```python
from build123d import *

# Parameters (mm, degrees)
SKETCH1_W           = 52
SKETCH1_H           = 53
BOSS_EXTRUDE1_DEPTH = 2
SKETCH2_W           = 48
SKETCH2_H           = 49
SKETCH2_W_2         = 44
SKETCH2_H_2         = 45
BOSS_EXTRUDE2_DEPTH = 5
CUT_EXTRUDE1_START  = -7
SKETCH3_W           = 4
SKETCH3_H           = 20
CUT_EXTRUDE1_DEPTH  = 7
FILLET1_R           = 2
SKETCH4_W           = 48
SKETCH4_H           = 2
CUT_EXTRUDE2_DEPTH  = 5


with BuildPart() as part:
    # Sketch1 → Boss-Extrude1 (new body)
    with BuildSketch(Plane.XY):
        with Locations((26, 26.5)):
            Rectangle(SKETCH1_W, SKETCH1_H)
    extrude(amount=BOSS_EXTRUDE1_DEPTH)

    # Sketch2 → Boss-Extrude2 (add)
    with BuildSketch(Plane.XY.offset(2)):
        with Locations((26, 26.5)):
            Rectangle(SKETCH2_W, SKETCH2_H)
        with Locations((26, 26.5)):
            Rectangle(SKETCH2_W_2, SKETCH2_H_2, mode=Mode.SUBTRACT)
    extrude(amount=BOSS_EXTRUDE2_DEPTH)

    # Sketch3 → Cut-Extrude1 (cut)
    with BuildSketch(Plane(origin=(0, 0, 0), x_dir=(-1, 0, 0), z_dir=(0, 0, -1)).offset(CUT_EXTRUDE1_START)):
        with Locations((-50, 25.5)):
            Rectangle(SKETCH3_W, SKETCH3_H)
    extrude(amount=CUT_EXTRUDE1_DEPTH, mode=Mode.SUBTRACT)

    # Fillet1
    fillet1_edges = [part.edges().sort_by_distance(p)[0] for p in [
        (48, 15.5, 1),
        (48, 35.5, 1),
    ]]
    fillet(fillet1_edges, radius=FILLET1_R)
    fillet1_2_edges = [part.edges().sort_by_distance(p)[0] for p in [
        (52, 15.5, 1),
        (52, 35.5, 1),
    ]]
    fillet(fillet1_2_edges, radius=FILLET1_R - 0.0001)  # a hair under: the kernel refuses the full size

    # Sketch4 → Cut-Extrude2 (cut)
    with BuildSketch(Plane.XY.offset(7)):
        with Locations((26, 3)):
            Rectangle(SKETCH4_W, SKETCH4_H)
    extrude(amount=-CUT_EXTRUDE2_DEPTH, mode=Mode.SUBTRACT)


solid = part.part
```
Verification items for the finished model (mm, model axes). A direction names the side the tool comes from. Round coordinates to 2 decimals unless told otherwise and drop trailing zeros. Order: outer loops, then holes, each group sorted by start corner. A loop starts at its lowest first (then second) coordinate and runs counter-clockwise, first axis right, second up. Notation, with made-up numbers: (25, -11) -> (57, -11) arc R6 cw to (57, -4) -> close; hole circle Ø2 at (-39.75, 26). An arc over 180 degrees is marked (long way). Put each result on its own line as item: value. Start each with the question number.
(1) Section check D-D (y = 29). Enter the section's corners in (x, z).
(2) Section check A-A (z = 5.25). Enter the section's corners in (x, y).
(3) Draft check along X on faces 5 (the face through (26, 49, 4)), 6 (the face through (26, 21, 2)), 7 (the face through (26, 51, 4)), 8 (the face through (0, 26, 1)). Enter one of: +X half, -X half, draft (parallel to the pull), parting line (faces both ways), or undercut.
(4) Section check B-B (y = 47). Enter the section's corners in (x, z).
(5) Material ranges on line 1 along X through (y, z) = (6.5, 4.5); line 2 along Z through (x, y) = (12.5, 3); line 3 along Y through (x, z) = (47, 5.5), recorded low to high.
(6) Section check C-C (x = 24). Enter the section's corners in (y, z).
(7) Tool access check on faces 1 (the face through (48, 42, 4)), 2 (the face through (2, 27, 4)), 3 (the face through (51.4, 36.07, 0.99)), 4 (the face through (49, 4, 5)). Record the directions out of +Z, -Z, +X, -X, +Y, -Y that give a thin tool (end or side, any length) a straight path to the whole face; none if there is none.
(8) Depth check by flat-ended pin: pin 1 Ø1 at (x, z) = (49, 3.5) entering from -Y; pin 2 Ø1.6 at (x, z) = (49, 4.5) entering from +Y; pin 3 Ø1.5 at (y, z) = (18.5, 4.5) entering from -X. Enter the tip coordinate at first touch or a pass-through.
Completed:
1. outline: (0, 0) -> (48, 0) -> (48, 2) -> (4, 2) -> (4, 7) -> (2, 7) -> (2, 2) -> (0, 2) -> close
2. outline: (2, 4) -> (4, 4) -> (4, 49) -> (48, 49) -> (48, 35.5) -> (50, 35.5) -> (50, 51) -> (2, 51) -> close; (48, 4) -> (50, 4) -> (50, 15.5) -> (48, 15.5) -> close
3. face 5: undercut
3. face 6: undercut
3. face 7: draft
3. face 8: -X half
4. outline: (0, 0) -> (52, 0) -> (52, 2) -> (50, 2) -> (50, 7) -> (48, 7) -> (48, 2) -> (4, 2) -> (4, 7) -> (2, 7) -> (2, 2) -> (0, 2) -> close
5. line 1: x = 2 to 4, 48 to 50
5. line 2: z = 0 to 2
5. line 3: y = 49 to 51
6. outline: (0, 0) -> (53, 0) -> (53, 2) -> (51, 2) -> (51, 7) -> (49, 7) -> (49, 2) -> (0, 2) -> close
7. face 1: +Z, -Y
7. face 2: +Z, -X, +Y, -Y
7. face 3: +Z, -Z, +X
7. face 4: +Z, +X, -X, -Y
8. pin 1: stops at y = 4
8. pin 2: stops at y = 51
8. pin 3: stops at x = 2
